For this review, take the finished solid that the model builds, in its own axes (mm). A direction names the side the tool comes from. Round coordinates to 2 decimals unless told otherwise and drop trailing zeros. Loops run counter-clockwise (first coordinate to the right, second up) from the corner with the lowest first, then second, coordinate; pieces in that order, holes last.
```python
from build123d import *

# Parameters (mm, degrees)
F0_W     = 14.25
F0_H     = 20.25
F1_DEPTH = 18
F2_W     = 20
F2_H     = 40
F3_DEPTH = 3
F4_R     = 1.775
F5_DEPTH = 20
F6_R     = 1.5


with BuildPart() as f1:
    # F0 (on Top) → F1 (new body)
    with BuildSketch(Plane.XY):
        Polygon((7.125, -10.125), (-7.125, -10.125), (0, -17.25), align=None)
        Polygon((0, 17.25), (-7.125, 10.125), (7.125, 10.125), align=None)
        Rectangle(F0_W, F0_H)
    extrude(amount=F1_DEPTH)

    # F2 (on Top) → F3 (join)
    with BuildSketch(Plane.XY):
        Rectangle(F2_W, F2_H)
    extrude(amount=F3_DEPTH)

    # F4 (on face) → F5 (join)
    with BuildSketch(Plane.XY.offset(18)):
        with Locations((0, 9.5)):
            Circle(F4_R)
        with Locations((0, -9.5)):
            Circle(F4_R)
    extrude(amount=F5_DEPTH)

    # F6
    f6_edges = [f1.edges().sort_by_distance(p)[0] for p in [
        (-1.775, -9.5, 38),
        (-1.775, 9.5, 38),
    ]]
    fillet(f6_edges, radius=F6_R)


solid = f1.part
```
(1) Insertion check: pin 1 Ø5 at (x, z) = (0.5, 34) entering from -Y (3 decimals); pin 2 Ø7 at (x, y) = (2, -7) entering from +Z; pin 3 Ø4 at (x, y) = (3, 6) entering from +Z; pin 4 Ø7.5 at (y, z) = (2, 13) entering from -X (3 decimals). Each pin has a flat end and moves straight along its axis. Give the tip position at first contact, or say it passes through.
(2) Add section C-C (x = -2.75). Give the boundary of the cut face in (y, z), plus the area to 3 significant figures.
(3) Add section B-B (z = 19.5). Give the boundary of the cut face in (x, y) (3 decimals).
(4) For faces 4 (the flat face through (3.61, 13.64, 10.4)), 5 (the cylindrical face through (-0.23, -7.74, 27.12)), 6 (the flat face through (-7.125, 0, 10)), 7 (the flat face through (-3.61, -13.64, 10.4)), list the 3-axis set-ups (+Z, -Z, +X, -X, +Y, -Y) from which the entire face can be reached by the end or side of a thin tool; tool diameter is ignored.
(5) The part is to be moulded in two halves that separate along Y. For faces 1 (the flat face through (3.51, -13.74, 10.4)), 2 (the flat face through (-3.51, 13.74, 10.4)), 3 (the cylindrical face through (-0.23, 11.26, 27.12)), say which applies: pulls with the +Y half, pulls with the -Y half, needs draft (parallel to the pull), parting line crosses it, or undercut.
(6) For L1, parallel to Y at x = 0, z = 32.5 (3 decimals); L2, parallel to Y at x = -1.25, z = 35; L3, parallel to Z at x = 9, y = 12.5, list the stretches that pass through material, from the lowest coordinate up.
(7) Add section A-A (y = 3). Give the boundary of the cut face in (x, z) (3 decimals), plus the area to 3 significant figures.
Outcome:
1. pin 1: stops at y = -11.275
1. pin 2: stops at z = 38
1. pin 3: stops at z = 18
1. pin 4: stops at x = -7.125
2. outline: (-20, 0) - (20, 0) - (20, 3) - (14.5, 3) - (14.5, 18) - (-14.5, 18) - (-14.5, 3) - (-20, 3) - close
2. area: 555 mm2
3. outline: circle Ø3.55 at (0, -9.5); circle Ø3.55 at (0, 9.5)
4. face 4: +Z, +X, +Y
4. face 5: +Z
4. face 6: +Z, -X, +Y, -Y
4. face 7: +Z, -X, -Y
5. face 1: pulls with the -Y half
5. face 2: pulls with the +Y half
5. face 3: undercut
6. L1: y = -11.275 to -7.725, 7.725 to 11.275
6. L2: y = -10.76 to -8.24, 8.24 to 10.76
6. L3: z = 0 to 3
7. outline: (-10, 0) - (10, 0) - (10, 3) - (7.125, 3) - (7.125, 18) - (-7.125, 18) - (-7.125, 3) - (-10, 3) - close
7. area: 274 mm2
